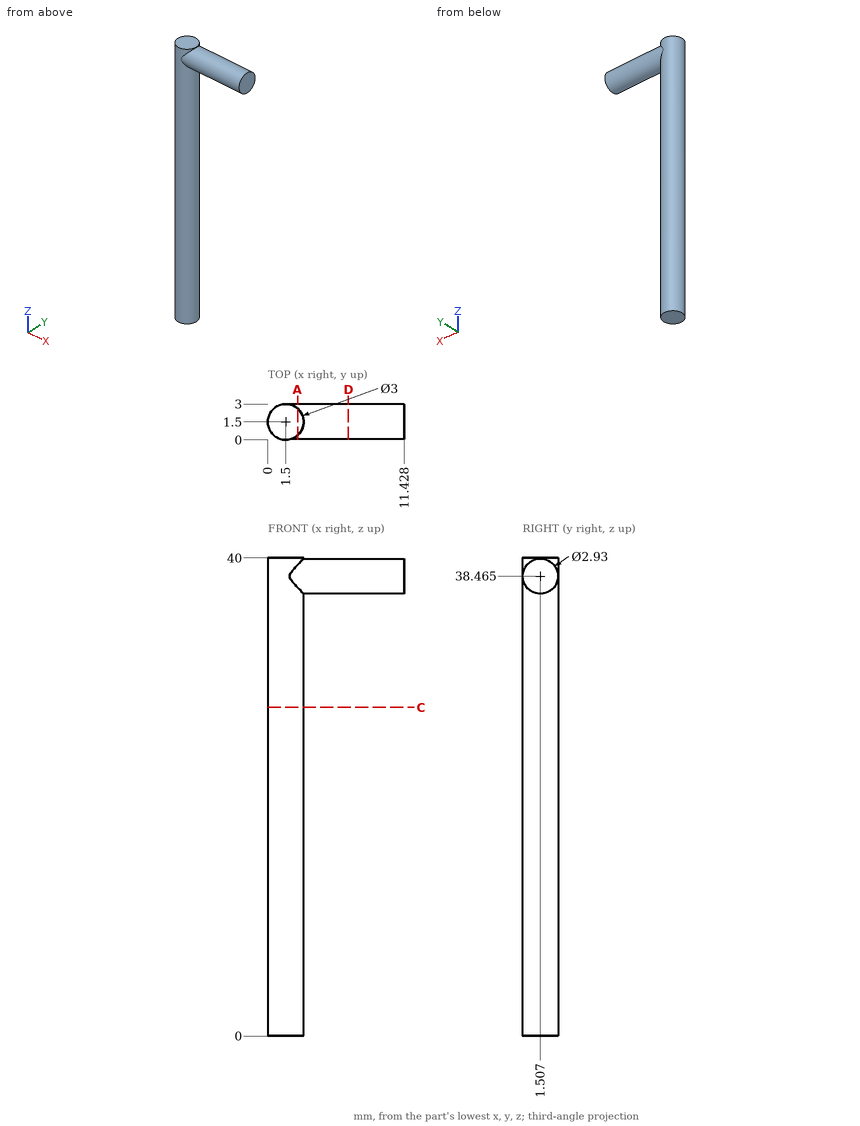
Drawing for the job (mm, zero at the part's lowest x, y, z). Give positions to 0.01 mm unless a question says otherwise; leave off trailing zeros. Order: outer loops, then holes, each group sorted by start corner. A loop starts at its lowest first (then second) coordinate and runs counter-clockwise, first axis right, second up. Notation, with made-up numbers: M 68.25,19.25 L 91.25,19.25 A8 cw 91.25,25.25 Z; hole C 8.25,17 d3. An arc over 180 degrees is marked long. Use a Markdown table: item, result. Add a question column.
(1) Saw through at A-A, the plane x = 2.5. Give the cut face in (y, z) (1 decimal).
(2) Drop flat-ended pins along their axis: P1, Ø2, axis at x = 3, z = 34, coming from the -Y side (1 decimal); P2, Ø1.5, axis at x = 8.5, y = 2.5, coming from the -Z side. Give the stop position or say it passes through.
(3) Saw through at D-D, the plane x = 6.75. Give the cut face in (y, z) (1 decimal).
(4) Probe line 1 along X through (y, z) = (1.65, 22); line 2 along X through (y, z) = (0.25, 5.5). List the from-to ranges inside material, lowest first. Write a range as [from, to].
(5) Saw through at C-C, the plane z = 27.5. Give the cut face in (x, y).
Answer key:
| question | item | result |
|---|---|---|
| 1 | outline | M 0.4,0 L 2.6,0 L 2.6,37.5 A1.5 ccw 2.6,39.4 L 2.6,40 L 0.4,40 L 0.4,39.4 A1.5 ccw 0.4,37.5 Z |
| 2 | P1 | y = 0.1 |
| 2 | P2 | z = 37.02 |
| 3 | outline | C 1.5,38.5 d2.9 |
| 4 | line 1 | [0.01, 2.99] |
| 4 | line 2 | [0.67, 2.33] |
| 5 | outline | C 1.5,1.5 d3 |
